Solid Edge part; units mm, degrees
sketch "Sketch1" plane through (0, 0, 0) normal (0, -1, 0) x (1, 0, 0)
  line L0 (-30, 3.5) -> (30, 3.5)
  line L1 (30, 3.5) -> (30, -3.5)
  line L2 (30, -3.5) -> (-30, -3.5)
  line L3 (-30, -3.5) -> (-30, 3.5)
  dimension "D1" = 30
  dimension "D2" = 30
extrude "Protrusion1" add sketch "Sketch1" against normal blind 70
sketch "Sketch2" plane through (0, 35, 3.5) normal (0, 0, 1) x (0, 1, 0)
  line L0 (15, 3.25) -> (-15, 3.25)
  line L1 (-15, 3.25) -> (-15, -3.25)
  line L2 (-15, -3.25) -> (15, -3.25)
  line L3 (15, -3.25) -> (15, 3.25)
  dimension "D1" = 15
  dimension "D2" = 15
extrude "Utskärning_för_vertikal_pelare" cut sketch "Sketch2" against normal blind 5
fillet "Avrundingar_15" radius 15 4 edges at (30, 70, 0) (-30, 70, 0) (-30, 0, 0) (30, 0, 0)
fillet "Avrundningar_1" radius 1 8 edges at (0, 70, 3.5) (-30, 35, 3.5) (30, 35, 3.5) (0, 0, 3.5) (-25.6066, 4.3934, 3.5) (25.6066, 4.3934, 3.5) (25.6066, 65.6066, 3.5) (-25.6066, 65.6066, 3.5)
sketch "Sketch3" plane through (0, 35, 3.5) normal (0, 0, 1) x (1, 0, 0)
  line L0 (-8.9011, -1.9226) -> (-8.9011, 1.9226)
  line L1 (-8.9011, 1.9226) -> (-15.9011, 1.9226)
  line L2 (-15.9011, 1.9226) -> (-15.9011, 3.9226)
  line L3 (-15.9011, 3.9226) -> (-21.6987, 0)
  line L4 (-21.6987, 0) -> (-15.9011, -3.9226)
  line L5 (-15.9011, -3.9226) -> (-15.9011, -1.9226)
  line L6 (-15.9011, -1.9226) -> (-8.9011, -1.9226)
  dimension "D1" = 15.9011
  dimension "D2" = 15.9011
  dimension "D3" = 8.9011
  dimension "D4" = 8.9011
extrude "Cutout1" cut sketch "Sketch3" against normal through all
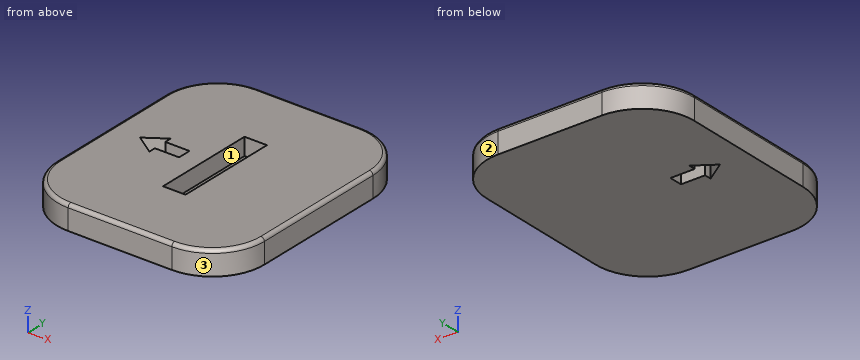
Read the model definition and answer for the solid it produces. Units are mm, in the model's axes. Face numbers are marked on the shaded views. Give positions to 0.01 mm unless a question says otherwise; leave off trailing zeros. Write each loop counter-clockwise with the first axis right and the second up, starting at its lowest first coordinate (ties: lowest second). Pieces come first, ordered by that corner, then holes. Notation, with made-up numbers: (-19.75, 49) - (15.25, 49) arc R8 ccw to (15.25, 53) - close; hole circle Ø8 at (-39, 38.5). An arc over 180 degrees is marked (long way). Answer in a Markdown table with one row per item. Add a question column.
Item 1: Section A-A, the plane z = -0.5 is taken. Write down the section's boundary in (x, y).
Item 2: Determine the mould class of the marked faces 1, 2 and 3 for opening direction Y: pulls with the +Y half, pulls with the -Y half, needs draft (parallel to the pull), parting line crosses it, or undercut.
Item 3: A flat-ended cylindrical pin translates along its axis: P1, Ø2, axis at x = 1, y = 30, coming from the +Z side. Find the tip coordinate at first contact, or state that the pin passes through.
Item 4: Section B-B, the plane y = 44 is taken. Write down the section's boundary in (x, z).
Item 5: Find the intervals of material crossed by L1, parallel to X at y = 43, z = 2.5; L2, parallel to Y at x = -0.5, z = 2; L3, parallel to X at y = 55.5, z = -1.5, in increasing order.
Recorded:
| question | item | result |
|---|---|---|
| 1 | outline | (-30, 15) arc R15 ccw to (-15, 0) - (15, 0) arc R15 ccw to (30, 15) - (30, 55) arc R15 ccw to (15, 70) - (-15, 70) arc R15 ccw to (-30, 55) - close; hole (-21.7, 35) - (-15.9, 31.08) - (-15.9, 33.08) - (-8.9, 33.08) - (-8.9, 36.92) - (-15.9, 36.92) - (-15.9, 38.92) - close; hole (-3.25, 20) - (3.25, 20) - (3.25, 50) - (-3.25, 50) - close |
| 2 | face 1 | undercut |
| 2 | face 2 | pulls with the +Y half |
| 2 | face 3 | pulls with the -Y half |
| 3 | P1 | stops at z = -1.5 |
| 4 | outline | (-30, -3.5) - (30, -3.5) - (30, 2.5) arc R1 ccw to (29, 3.5) - (3.25, 3.5) - (3.25, -1.5) - (-3.25, -1.5) - (-3.25, 3.5) - (-29, 3.5) arc R1 ccw to (-30, 2.5) - close |
| 5 | L1 | x = -30 to -3.25, 3.25 to 30 |
| 5 | L2 | y = 0 to 20, 50 to 70 |
| 5 | L3 | x = -29.99 to 29.99 |
